Autodesk Inventor part; units mm, degrees
ref_plane "作業平面1" through (0, -10, 10.934005) normal (0, 1, 0) x (-1, 0, 0)
ref_plane "YZ Plane" through (0, 0, 0) normal (1, 0, 0) x (0, 1, 0)
ref_plane "XY Plane" through (0, 0, 0) normal (0, 0, 1) x (1, 0, 0)
sketch "スケッチ1" plane through (0, 0, 0) normal (1, 0, 0) x (0, 1, 0)
  line L0 (0, -9.065995) -> (0, 0.934005)
  line L1 (0, 0) -> (12.5, 0)
  line L2 (12.5, 0) -> (12.5, -2.385786)
  line L3 (12.5, -2.385786) -> (10.5, -3.060246)
  line L4 (10.5, -3.060246) -> (10.5, -5.803392)
  line L5 (10.5, -5.803392) -> (12.5, -6.680209)
  line L6 (12.5, -6.680209) -> (12.5, -9.065995)
  line L7 (12.5, -9.065995) -> (0, -9.065995)
  line L8 (0, -9.065995) -> (0, 0)
  line L9 (10.5, -4.431819) -> (0, -4.532998)
  line L10 (10.5, -27.060246) -> (10.5, -29.803392)
  line L11 (12.5, -30.680209) -> (12.5, -33.065995)
  line L12 (10.5, -29.803392) -> (12.5, -30.680209)
  line L13 (12.5, -26.385786) -> (10.5, -27.060246)
  line L14 (12.5, -24) -> (12.5, -26.385786)
  line L15 (0, -24) -> (12.5, -24)
  line L16 (12.5, -33.065995) -> (0, -33.065995)
  line L17 (10.5, -28.431819) -> (0, -28.532998)
  line L18 (0, -33.065995) -> (0, -23.065995)
  line L19 (0, -33.065995) -> (0, -24)
  line L20 (10.5, -51.060246) -> (10.5, -53.803392)
  line L21 (12.5, -54.680209) -> (12.5, -57.065995)
  line L22 (10.5, -53.803392) -> (12.5, -54.680209)
  line L23 (12.5, -50.385786) -> (10.5, -51.060246)
  line L24 (12.5, -48) -> (12.5, -50.385786)
  line L25 (0, -48) -> (12.5, -48)
  line L26 (12.5, -57.065995) -> (0, -57.065995)
  line L27 (10.5, -52.431819) -> (0, -52.532998)
  line L28 (0, -57.065995) -> (0, -47.065995)
  line L29 (0, -57.065995) -> (0, -48)
  line L30 (10.5, -75.060246) -> (10.5, -77.803392)
  line L31 (12.5, -78.680209) -> (12.5, -81.065995)
  line L32 (10.5, -77.803392) -> (12.5, -78.680209)
  line L33 (12.5, -74.385786) -> (10.5, -75.060246)
  line L34 (12.5, -72) -> (12.5, -74.385786)
  line L35 (0, -72) -> (12.5, -72)
  line L36 (12.5, -81.065995) -> (0, -81.065995)
  line L37 (10.5, -76.431819) -> (0, -76.532998)
  line L38 (0, -81.065995) -> (0, -71.065995)
  line L39 (0, -81.065995) -> (0, -72)
  line L40 (0, -81.065995) -> (12.5, -81.065995)
  line L41 (12.5, -81.065995) -> (12.5, -86.473236)
  line L42 (12.5, -86.473236) -> (0, -86.473236)
  line L43 (0, -86.473236) -> (0, -81.065995)
  line L44 (12.5, -72) -> (12.5, -57.065995)
  line L45 (12.5, -48) -> (12.5, -33.065995)
  line L46 (12.5, -24) -> (12.5, -9.065995)
  line L47 (0, 0) -> (12.5, 0)
  line L48 (12.5, 0) -> (12.5, 5.934005)
  line L49 (12.5, 5.934005) -> (0, 5.934005)
  line L50 (0, 5.934005) -> (0, 0)
  line L51 (0, 5.934005) -> (10, 5.934005)
  line L52 (10, 5.934005) -> (10, 15.934005)
  line L53 (10, 15.934005) -> (0, 15.934005)
  line L54 (0, 15.934005) -> (0, 5.934005)
  line L55 (0, 15.934005) -> (0, -71.065995)
  circle A0 centre (12.5, -4.496449) radius 2
  point P0 (0, 0)
  point P1 (6.25, -86.473236)
  point P2 (0, -4.065995)
  point P3 (0, 0)
  point P4 (0, -23.065995)
  point P5 (0, -33.065995)
  point P6 (0, -47.065995)
  point P7 (0, -57.065995)
  point P8 (10, 5.934005)
  dimension "d1" = 2.74315
  dimension "d2" = 12.5
  dimension "d7" = 12.5
  dimension "d8" = 10
  dimension "d9" = 2.38579
  dimension "d10" = 2.38579
  dimension "d11" = 90
  dimension "d12" = 90
  dimension "d13" = 90
  dimension "d14" = 0
  dimension "d17" = 24
  dimension "d22" = 10
  dimension "d23" = 0
  dimension "d24" = 0
  dimension "d25" = 10
  dimension "d26" = 10
  dimension "d27" = 10
  dimension "d44" = 4
  dimension "d45" = 10.5
  dimension "d46" = 108.636
sketch "スケッチ1 outline for 回転1" plane through (0, 0, 0) normal (1, 0, 0) x (0, 1, 0)
  line L0 (10, 15.934005) -> (0, 15.934005)
  line L1 (10, 5.934005) -> (10, 15.934005)
  line L2 (12.5, 5.934005) -> (10, 5.934005)
  line L3 (12.5, 0) -> (12.5, 5.934005)
  line L4 (12.5, -2.385786) -> (12.5, 0)
  line L5 (10.5, -3.060246) -> (12.5, -2.385786)
  line L6 (10.5, -5.803392) -> (10.5, -3.060246)
  line L7 (12.5, -6.680209) -> (10.5, -5.803392)
  line L8 (12.5, -9.065995) -> (12.5, -6.680209)
  line L9 (12.5, -24) -> (12.5, -9.065995)
  line L10 (12.5, -26.385786) -> (12.5, -24)
  line L11 (10.5, -27.060246) -> (12.5, -26.385786)
  line L12 (10.5, -29.803392) -> (10.5, -27.060246)
  line L13 (12.5, -30.680209) -> (10.5, -29.803392)
  line L14 (12.5, -33.065995) -> (12.5, -30.680209)
  line L15 (12.5, -48) -> (12.5, -33.065995)
  line L16 (12.5, -50.385786) -> (12.5, -48)
  line L17 (10.5, -51.060246) -> (12.5, -50.385786)
  line L18 (10.5, -53.803392) -> (10.5, -51.060246)
  line L19 (12.5, -54.680209) -> (10.5, -53.803392)
  line L20 (12.5, -57.065995) -> (12.5, -54.680209)
  line L21 (12.5, -72) -> (12.5, -57.065995)
  line L22 (12.5, -74.385786) -> (12.5, -72)
  line L23 (10.5, -75.060246) -> (12.5, -74.385786)
  line L24 (10.5, -77.803392) -> (10.5, -75.060246)
  line L25 (12.5, -78.680209) -> (10.5, -77.803392)
  line L26 (12.5, -81.065995) -> (12.5, -78.680209)
  line L27 (12.5, -86.473236) -> (12.5, -81.065995)
  line L28 (0, -86.473236) -> (12.5, -86.473236)
  line L29 (0, -81.065995) -> (0, -86.473236)
  line L30 (0, -71.065995) -> (0, -81.065995)
  line L31 (0, -57.065995) -> (0, -71.065995)
  line L32 (0, -47.065995) -> (0, -57.065995)
  line L33 (0, -33.065995) -> (0, -47.065995)
  line L34 (0, -23.065995) -> (0, -33.065995)
  line L35 (0, -9.065995) -> (0, -23.065995)
  line L36 (0, 0) -> (0, -9.065995)
  line L37 (0, 5.934005) -> (0, 0)
  line L38 (0, 15.934005) -> (0, 5.934005)
revolve "回転1" add sketch "スケッチ1 outline for 回転1" angle 360 about axis through (0, 0, 15.934005) along (0, 0, -1)
sketch "スケッチ2" plane through (0, 0, -86.473236) normal (0, 0, -1) x (-1, 0, 0)
  circle A0 centre (0, 0) radius 5.2
  point P0 (0, 0)
  dimension "d29" = 10.4
extrude "押し出し1" cut sketch "スケッチ2" against normal through all
ref_plane "作業平面1" through (0, -10, 10.934005) normal (0, 1, 0) x (-1, 0, 0)
sketch "スケッチ3" plane through (0, -10, 10.934005) normal (0, 1, 0) x (-1, 0, 0)
  line L0 (-10, 5) -> (10, 5)
  point P0 (0, -10.934005)
  point P1 (0, 0)
  dimension "d32" = 5
hole "穴1" at (0, -10, 10.934005) direction (0, 1, 0) diameter 3.4 end through all
sketch "スケッチ4" plane through (0, 0, 15.934005) normal (0, 0, 1) x (1, 0, 0)
  circle A0 centre (0, 0) radius 10
  line L0 (5, -8.660254) -> (-5, -8.660254)
  line L1 (10, 0) -> (-10, 0)
  line L2 (5, 8.660254) -> (-5, 8.660254)
  point P0 (0, 0)
  dimension "d40" = 10
  dimension "d41" = 20
extrude "押し出し2" cut sketch "スケッチ4" against normal blind 10 contours L2 A0 | A0 L0
properties part number "ball_loading_v1_3DP_P_B" material "ABS プラスチック"
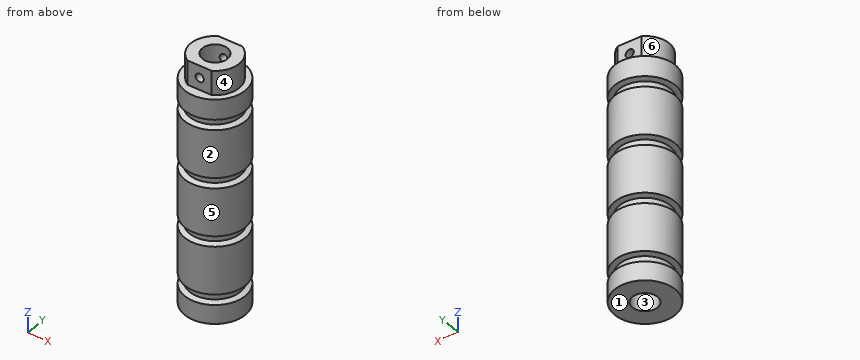
Could you check a few things on this model? Use its own coordinates, in mm. Face numbers are marked on the shaded views. A direction names the side the tool comes from. Coordinates: 2 decimals unless noted, no trailing zeros. Order: outer loops, then holes, each group sorted by start corner. A loop starts at its lowest first (then second) coordinate and runs counter-clockwise, first axis right, second up.
Q1. Which directions (+Z, -Z, +X, -X, +Y, -Y) give clear straight access to the entire face, cutting with the end or side of a thin tool? Please do the marked faces 4, 5 and 6.
Q2. Will these pins go through, and if not, where does the flat tip stop? pin 1 (6 mm diameter, centred on y = 7.5, z = -55.5, fed in from +X); pin 2 (3 mm diameter, centred on x = 10, y = -5, fed in from +Z); pin 3 (1.5 mm diameter, centred on y = -7.5, z = -70.5, fed in from +X); pin 4 (6 mm diameter, centred on y = -8.5, z = -25.5, fed in from +X) (3 decimals).
Q3. Suppose I cut it at A-A on z = -64. Please give me the cut outline in (x, y).
Q4. Thinking about a two-plate mould opening in Y: for the marked faces 1, 2 and 3, which applies, released by +Y, released by -Y, zero draft, split by the parting line, or undercut?
Q5. Please list where these lines run through material, in increasing order: L1, parallel to Z at x = 0, y = 7.3; L2, parallel to Y at x = -7.5, z = -49.5; L3, parallel to Y at x = 2.75, z = -75.5.
Q6. Suppose I cut it at B-B on x = 0. Give the number of separate pieces and of enclosed holes in the cut face, and give its area (3 significant figures).
Answer:
1. face 4: +Z, +X
1. face 5: +Z, -Z
1. face 6: +Z, -X
2. pin 1: stops at x = 11.66
2. pin 2: stops at z = 15.93
2. pin 3: stops at x = 10.52
2. pin 4: stops at x = 11.225
3. outline: circle Ø25 at (0, 0); hole circle Ø10.4 at (0, 0)
4. face 1: zero draft
4. face 2: split by the parting line
4. face 3: undercut
5. L1: z = -86.47 to 9.23, 12.63 to 15.93
5. L2: y = -10 to 10
5. L3: y = -10.13 to -4.41, 4.41 to 10.13
6. separate pieces: 4
6. enclosed holes: 0
6. area: 1,340 mm2
